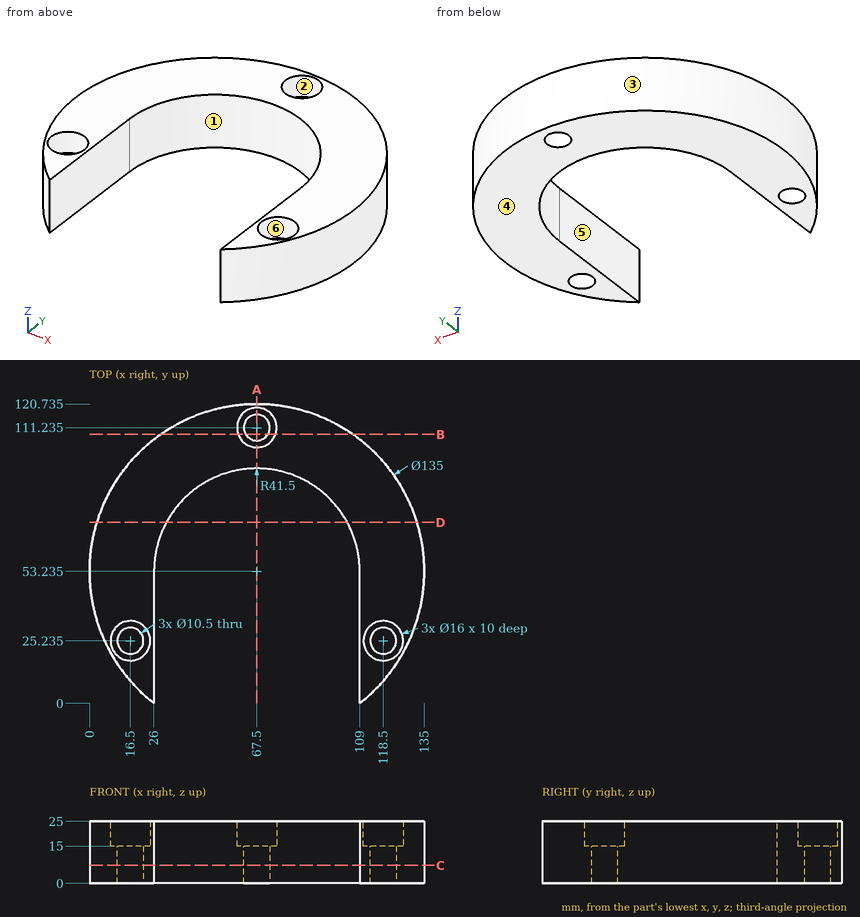
Geometry: see drawing. Coordinates: mm, zero at the bounding-box minimum. A direction names the side the tool comes from. Give positions to 0.01 mm unless a question says otherwise; leave off trailing zeros. Write each loop counter-clockwise with the first axis right and the second up, starting at its lowest first coordinate (ties: lowest second). Pieces come first, ordered by that corner, then holes. Notation, with made-up numbers: (44, 67) - (68, 67) arc R22 cw to (68, 93) - close; hole circle Ø11 at (11, 64.25). An arc over 180 degrees is marked (long way). Return JSON: item names as keys, results as strings. Group by question number.
1) First-contact query: P1, Ø13, axis at x = 15.5, y = 26, coming from the +Z side; P2, Ø18.5, axis at x = 67.5, y = 111.24, coming from the -Z side; P3, Ø2, axis at x = 84.5, z = 20.5, coming from the +Y side; P4, Ø3, axis at y = 63, z = 12.5, coming from the -X side. Flat tips, straight axial feed; report the tip coordinate or a pass-through.
2) Line query: line 1 (X direction, y = 22.5, z = 14.5); line 2 (Y direction, x = 67.5, z = 11.25) (1 decimal); line 3 (X direction, y = 62.5, z = 13.25). Output: solid intervals per line, ascending.
3) Mould query, pull axis Y, two halves, no side actions, for the marked faces 1, 2 and 3. Classes: released by +Y, released by -Y, zero draft, split by the parting line, or undercut.
4) Set-up query: the marked faces 4, 5 and 6. Return all of +Z, -Z, +X, -X, +Y, -Y with unobstructed straight access to the full face (end or side cutting, diameter ignored); none if empty.
5) Section C-C on z = 7.25. State how many separate pieces and enclosed holes the cut face has, plus the area to 3 significant figures.
6) Section D-D on y = 73. Return the cut outline in (x, z).
7) Section B-B on y = 108.5. Return the cut outline in (x, z), plus the area to 3 significant figures.
8) Section A-A on x = 67.5. Return the cut outline in (y, z) (1 decimal).
Filled in:
{
 "1": {"P1": "stops at z = 15", "P2": "stops at z = 0", "P3": "stops at y = 118.81", "P4": "stops at x = 0.51"},
 "2": {"line 1": "x = 7.4 to 12.02, 20.98 to 26, 109 to 114.02, 122.98 to 127.6", "line 2": "y = 94.7 to 106, 116.5 to 120.7", "line 3": "x = 0.64 to 27.05, 107.95 to 134.36"},
 "3": {"face 1": "released by -Y", "face 2": "undercut", "face 3": "split by the parting line"},
 "4": {"face 4": "-Z, +X, -X, +Y, -Y", "face 5": "+Z, -Z, -Y", "face 6": "+Z"},
 "5": {"separate pieces": "1", "enclosed holes": "3", "area": "6,120 mm^2"},
 "6": {"outline": "(2.96, 0) - (31.01, 0) - (31.01, 25) - (2.96, 25) - close; (103.99, 0) - (132.04, 0) - (132.04, 25) - (103.99, 25) - close"},
 "7": {"outline": "(28.74, 0) - (63.02, 0) - (63.02, 15) - (59.98, 15) - (59.98, 25) - (28.74, 25) - close; (71.98, 0) - (106.26, 0) - (106.26, 25) - (75.02, 25) - (75.02, 15) - (71.98, 15) - close", "area": "1,650 mm^2"},
 "8": {"outline": "(94.7, 0) - (106, 0) - (106, 15) - (103.2, 15) - (103.2, 25) - (94.7, 25) - close; (116.5, 0) - (120.7, 0) - (120.7, 25) - (119.2, 25) - (119.2, 15) - (116.5, 15) - close"}
}
